Source: CAD feature listing. Evaluate the final solid. Frame: model axes, mm. A direction names the side the tool comes from. Round coordinates to 2 decimals unless told otherwise and drop trailing zeros. Loops run counter-clockwise (first coordinate to the right, second up) from the corner with the lowest first, then second, coordinate; pieces in that order, holes last. Notation, with made-up numbers: M -33,-38.5 L -28,-38.5 A37 ccw -28,-2.5 Z; hole C 89,-28 d10. An arc over 180 degrees is marked long. One line per item, written item: value.
Autodesk Inventor part; units mm, degrees
ref_plane "Work Plane1" through (29, 0, 0) normal (0, -1, 0) x (1, 0, 0)
ref_plane "YZ Plane" through (0, 0, 0) normal (1, 0, 0) x (0, 1, 0)
ref_plane "XZ Plane" through (0, 0, 0) normal (0, 1, 0) x (-1, 0, 0)
sketch "Sketch1" plane through (0, 0, 0) normal (0, 0, 1) x (1, 0, 0)
  line L0 (-0.0931, 0) -> (6.35, 0)
  line L1 (6.35, 0) -> (6.35, 2.0828)
  line L2 (6.35, 2.0828) -> (1.5902, 2.0828)
  line L3 (1.5902, 2.0828) -> (0.0001, 2.0828)
  line L4 (0.0001, 2.0828) -> (0, 2.0828)
  line L5 (0, 2.0828) -> (0, 3.9624)
  line L6 (0, 3.9624) -> (-2.2098, 3.9624)
  line L7 (-2.2098, 3.9624) -> (-2.2098, 1.3785)
  line L8 (-2.2098, 1.3785) -> (-0.889, 1.3785)
  line L9 (-0.889, 1.3785) -> (-0.0931, 0)
  line L10 (-3.9218, 0) -> (8.062, 0)
  line L11 (0, -0.7925) -> (0, 4.7549)
  line L12 (1.5902, 2.0828) -> (0, 2.0828) construction
  dimension "d1" = 4.7598
  dimension "d2" = 1.5901
  dimension "d3" = 2.2098
  dimension "d4" = 1.3208
  dimension "d5" = 60
  dimension "d6" = 4.1656
  dimension "d7" = 4.1656
  dimension "d8" = 2.757
  dimension "d9" = 7.9248
  dimension "d26" = 6.35
revolve "Body" add sketch "Sketch1" angle 360 about axis through (-0.0931, 0, 0) along (1, 0, 0)
sketch "Sketch2" plane through (-2.2098, 0, 0) normal (-1, 0, 0) x (0, 0, 1)
  circle A0 centre (0, 0) radius 1.3785
  line L0 (0, -5.5474) -> (0, 5.5474)
  line L1 (-5.5474, 0) -> (5.5474, 0)
  line L2 (1.3785, 0) -> (0.6892, -1.1938)
  line L3 (0.6892, -1.1938) -> (-0.6892, -1.1938)
  line L4 (-0.6892, -1.1938) -> (-1.3785, 0)
  line L5 (-1.3785, 0) -> (-0.6892, 1.1938)
  line L6 (-0.6892, 1.1938) -> (0.6892, 1.1938)
  line L7 (0.6892, 1.1938) -> (1.3785, 0)
extrude "Slot" add sketch "Sketch2" against normal up to next contours L7 A0 | A0 L2 | L6 L0 A0 | A0 L0 L3 | L0 L6 A0 | A0 L3 L0 | L4 A0 | A0 L5
fillet "Fillet1" radius 1.9558 1 edges at (-2.2098, -3.9624, 0)
thread "Thread"
chamfer "Chamfer1" distance 0.4869 distance2 0.4869 1 edges at (6.35, -2.0828, 0) measured on face at (6.35, -0.5197, -0.4604)
ref_plane "Work Plane1" through (29, 0, 0) normal (0, -1, 0) x (1, 0, 0)
fillet "Fillet2" radius 0.1 1 edges at (0.0001, -2.0828, 0)
equation "\"d1\" = GEL"
equation "\"d3\" = KOH"
equation "\"d4\" = INTI"
equation "\"d6\" = GD"
equation "\"d7\" = BDM"
equation "\"d8\" = 1.1547 * SW"
equation "\"d9\" = KOD"
equation "\"d26\" = NLG"
equation "\"d30\" = R"
equation "\"d17\" = RR"
equation "\"d13\" = GEL"
equation "\"d15\" = -0.5 * SPD + 0.5 * GD"
equation "\"d16\" = GUL"
equation "\"GD\" = NND"
equation "\"NLG\" = 6.35"
equation "\"GEL\" = 4.75976"
equation "\"KOD\" = 7.9248"
equation "\"KOH\" = 2.2098"
equation "\"INTI\" = 1.3208"
equation "\"GAL\" = 1.59004"
equation "\"GUL\" = 0.48692"
equation "\"BDM\" = NND"
equation "\"SW\" = 2.3876"
equation "\"RR\" = 1.9558"
equation "\"SPD\" = 3.19176"
equation "\"R\" = 0.1"
equation "\"TOA\" = 30deg"
equation "\"GD1\" = SPD"
equation "\"THREADDIA\" = 4.1656"
equation "\"KOH1\" = 0.381"
equation "\"NND\" = 4.1656"
equation "\"E0\" = 2.75768"
properties part number "ANSI B18.3 - 8 - 32 x 1/4" material "Steel, Mild"
1. Pull-direction query (Y, two-part tool) for faces 3 (the face through (2.941, 1.987, -0.626)), 4 (the face through (6.35, 0, 0)), 5 (the face through (-2, -1.194, 0)); classes: released by +Y, released by -Y, zero draft, split by the parting line, or undercut.
Report:
face 3: split by the parting line
face 4: zero draft
face 5: undercut
2. Ray query, line 1 (Z direction, x = 2, y = 0); line 2 (Y direction, x = 2, z = -1.5). Return the intervals inside material, ascending. Write a range as [from, to].
Report:
line 1: z = [-2.08, 2.08]
line 2: y = [-1.45, 1.45]
3. Pin query (flat end, axial travel): pin 1 (0.7 mm diameter, centred on x = -1.5, z = 0, fed in from -Y); pin 2 (3 mm diameter, centred on y = 2.5, z = -1.5, fed in from -X); pin 3 (1.5 mm diameter, centred on x = -1.5, z = 0, fed in from +Y). Return the tip coordinate at first contact, or that it passes through.
Report:
pin 1: stops at y = -3.75
pin 2: stops at x = -2.21
pin 3: stops at y = 3.9
4. Section query C-C (x = -0.5). Return the cut outline in (y, z), and give its area (3 significant figures).
Report:
outline: C 0,0 d7.89; hole C 0,0 d1.41
area: 47.4 mm2
5. Reachability of faces 1 (the face through (-2.21, -1, -1)), 2 (the face through (-1.51, -0.59, 1.04)) from +Z, -Z, +X, -X, +Y, -Y: full face, straight path, thin tool, end or side. Return the list, or none.
Report:
face 1: +Z, -Z, -X, +Y, -Y
face 2: -X
6. Section query A-A (x = -1.5). Return the cut outline in (y, z), and give its area (3 significant figures).
Report:
outline: C 0,0 d7.03; hole M -1.19,-0.69 L 0,-1.38 L 1.19,-0.69 L 1.19,0.69 L 0,1.38 L -1.19,0.69 Z
area: 33.9 mm2
7. Section query B-B (x = 1.5). Return the cut outline in (y, z), and give its area (3 significant figures).
Report:
outline: C 0,0 d4.17
area: 13.6 mm2
